The listing builds one solid part. Answer for the finished solid, in the listing's coordinates (mm). Round coordinates to 2 decimals unless told otherwise and drop trailing zeros. Write each loop counter-clockwise with the first axis right and the second up, starting at its lowest first coordinate (ties: lowest second). Pieces come first, ordered by that corner, then holes. Notation, with made-up numbers: M 7,55 L 49,55 A29 cw 49,91 Z; hole C 83,73 d6. An arc over 180 degrees is marked long. Answer as CSV lines item,"result". Start each with the question number.
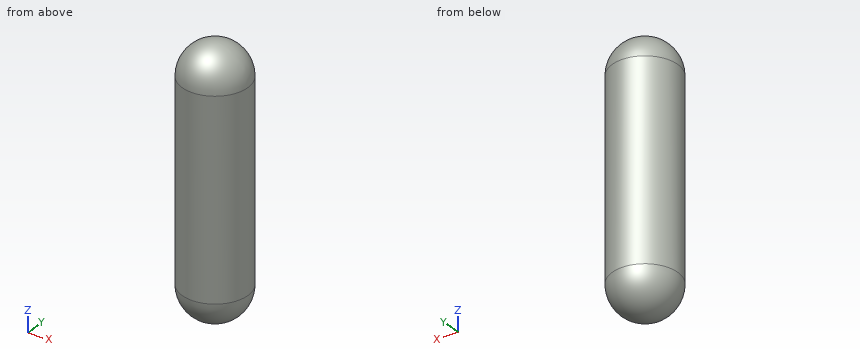
from build123d import *

# Parameters (mm, degrees)
F0_R     = 12.5
F1_DEPTH = 50
F2_R     = 12.5


with BuildPart() as f1:
    # F0 (on Top) → F1 (new body)
    with BuildSketch(Plane.XY):
        Circle(F0_R)
    extrude(amount=F1_DEPTH)

    # F2
    f2_edges = [f1.edges().sort_by_distance(p)[0] for p in [
        (-12.5, 0, 50),
    ]]
    fillet(f2_edges, radius=F2_R)

    # F3: F1 across plane


with BuildPart() as f1_1:
    add(f1.part)
    add(f1.part.mirror(Plane.XY))


solid = f1_1.part
Q1. Each of these flat-tipped pins is pushed along its axis until it touches: P1, Ø4, axis at x = -6.5, z = -16.5, coming from the -Y side; P2, Ø1.5, axis at y = -1.5, z = 32, coming from the +X side; P3, Ø4, axis at x = -1, y = -4, coming from the -Z side. Where does it stop, or does it pass through?
Q2. Straight lines are drawn through the part: L1, parallel to X at y = 2.5, z = -11; L2, parallel to Y at x = -6, z = -45; L3, parallel to Y at x = -6.25, z = -36. For each, find the intervals that lie inside material, in ascending order.
Q3. Find section C-C (z = -15). Determine the outline of the cut face in (x, y), plus the area to 3 significant figures.
Q4. Find section A-A (x = 0). Determine the outline of the cut face in (y, z).
Reported:
1,P1,"stops at y = -11.66"
1,P2,"stops at x = 12.48"
1,P3,"stops at z = -49.82"
2,L1,"x = -12.25 to 12.25"
2,L2,"y = -8 to 8"
2,L3,"y = -10.83 to 10.83"
3,outline,"C 0,0 d25"
3,area,"491 mm2"
4,outline,"M -12.5,-37.5 A12.5 ccw 12.5,-37.5 L 12.5,37.5 A12.5 ccw -12.5,37.5 Z"
